Could you check a few things on this drawing? It's one solid part, dimensions in mm from its lowest x, y, z. A direction names the side the tool comes from. Give positions to 0.01 mm unless a question says otherwise; leave off trailing zeros. Order: outer loops, then holes, each group sorted by start corner. A loop starts at its lowest first (then second) coordinate and runs counter-clockwise, first axis right, second up. Notation, with made-up numbers: (12, 10) -> (69, 10) arc R18 cw to (69, 25) -> close; hole circle Ø9 at (6.25, -27.5). An arc over 180 degrees is marked (long way). Answer as a JSON object with one key per item and string values.
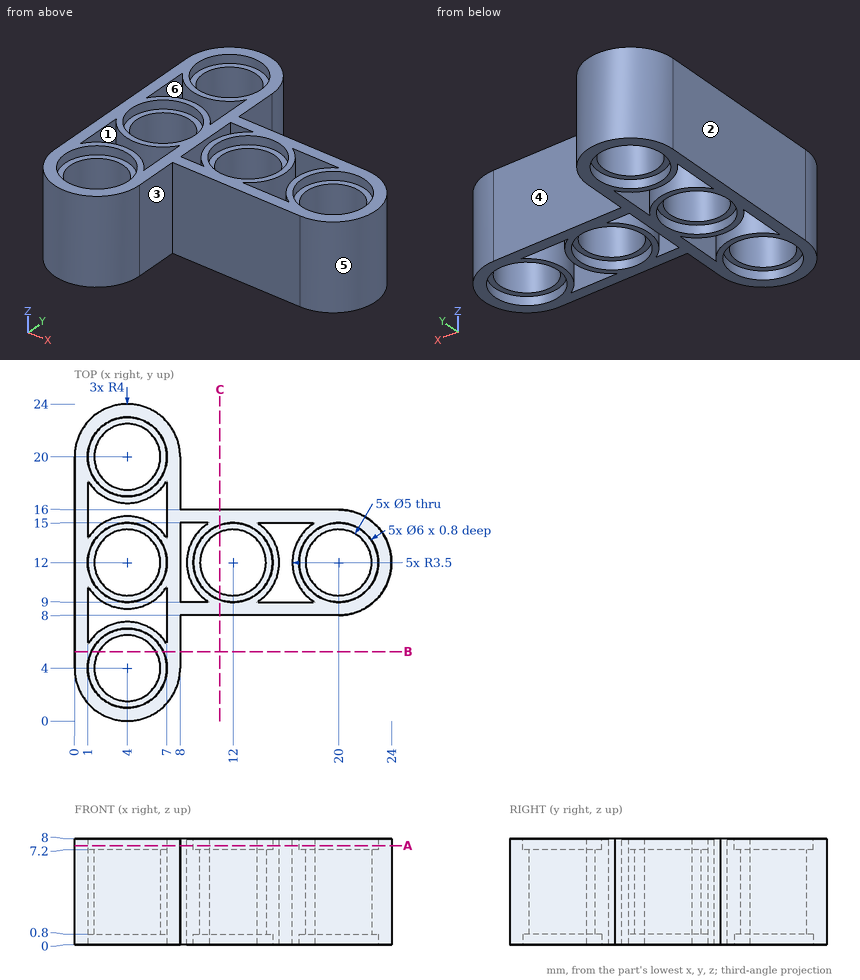
1. If we section it at B-B on y = 5.25: Please give me the cut outline in (x, z), then the cut area to 3 significant figures.
Worked answers:
{"outline": "(0, 0) -> (1.27, 0) -> (1.27, 0.8) -> (1.83, 0.8) -> (1.83, 7.2) -> (1.27, 7.2) -> (1.27, 8) -> (0, 8) -> close; (6.17, 0.8) -> (6.73, 0.8) -> (6.73, 0) -> (8, 0) -> (8, 8) -> (6.73, 8) -> (6.73, 7.2) -> (6.17, 7.2) -> close", "area": "27.6 mm²"}
2. Please list where these lines run through material, in increasing order: L1, parallel to Y at x = 12, z = 4; L2, parallel to Y at x = 20, z = 0.65; L3, parallel to X at y = 7, z = 1.25.
Worked answers:
{"L1": "8 to 9.5, 14.5 to 16", "L2": "8 to 9, 15 to 16", "L3": "0 to 1, 2.2 to 5.8, 7 to 8"}
3. Will these pins go through, and if not, where does the flat tip stop? pin 1 Ø4 at (x, z) = (16.5, 6) entering from -Y; pin 2 Ø3.5 at (x, y) = (12, 12) entering from -Z; pin 3 Ø1.5 at (x, z) = (6.5, 5) entering from -Y; pin 4 Ø1.8 at (x, y) = (5.5, 11) entering from -Z.
Worked answers:
{"pin 1": "y = 8", "pin 2": "through", "pin 3": "y = 0.4", "pin 4": "z = 0.8"}
4. If we section it at C-C on x = 11: Please give me the cut outline in (y, z), then the cut area to 3 significant figures.
Worked answers:
{"outline": "(8, 0) -> (9.17, 0) -> (9.17, 0.8) -> (9.71, 0.8) -> (9.71, 7.2) -> (9.17, 7.2) -> (9.17, 8) -> (8, 8) -> close; (14.29, 0.8) -> (14.83, 0.8) -> (14.83, 0) -> (16, 0) -> (16, 8) -> (14.83, 8) -> (14.83, 7.2) -> (14.29, 7.2) -> close", "area": "25.6 mm²"}
5. For the marked faces 4, 5 and 6, which set-ups out of +Z, -Z, +X, -X, +Y, -Y let a thin tool reach every point of the face, with its end or its side?
Worked answers:
{"face 4": "+Z, -Z, +X, +Y", "face 5": "+Z, -Z, +X", "face 6": "+Z, -Z"}
6. If we mould it in two halves opening along X, with no side actions, what happens to the marked faces 1, 2 and 3? For each: +X half, -X half, draft (parallel to the pull), parting line (faces both ways), or undercut.
Worked answers:
{"face 1": "undercut", "face 2": "-X half", "face 3": "+X half"}
7. If we section it at A-A on z = 7.5: Count the separate pieces of the cut face and the enclosed holes in it, then the cut area to 3 significant figures.
Worked answers:
{"separate pieces": "1", "enclosed holes": "9", "area": "116 mm²"}
